```python
from build123d import *

# Parameters (mm, degrees)
SKETCH_1_R      = 4.402451684
SKETCH_1_R_2    = 1.6
EXTRUDE_1_DEPTH = 2
EXTRUDE_4_DEPTH = 8.8


with BuildPart() as part:
    # 草图1 → 凸台-拉伸1 (new body)
    # profile 1 of 2: a face of its own
    with BuildSketch(Plane.XY):
        Circle(SKETCH_1_R)
        Circle(SKETCH_1_R_2, mode=Mode.SUBTRACT)
    # profile 2 of 2: a face of its own
    with BuildSketch(Plane.XY):
        with BuildLine():
            ThreePointArc((4.402451684, 0), (0, -4.402451684), (-4.402451684, 0))
            Line((-4.402451684, 0), (-4.402451684, -12.835731795))
            Line((-4.402451684, -12.835731795), (4.402451684, -12.835731795))
            Line((4.402451684, -12.835731795), (4.402451684, 0))
        make_face()
    extrude(amount=EXTRUDE_1_DEPTH)

    # 草图4 → 凸台-拉伸4 (add)
    with BuildSketch(Plane.ZY.offset(4.402451684)):
        with BuildLine():
            ThreePointArc((6, -8.835731795), (4.828427125, -6.00730467), (2, -4.835731795))
            Line((2, -4.835731795), (2, -5.835731795))
            ThreePointArc((2, -5.835731795), (4.121320344, -6.714411452), (5, -8.835731795))
            ThreePointArc((5, -8.835731795), (4.121320344, -10.957052139), (2, -11.835731795))
            Line((2, -11.835731795), (2, -12.835731795))
            ThreePointArc((2, -12.835731795), (4.828427125, -11.66415892), (6, -8.835731795))
        make_face()
    extrude(amount=-EXTRUDE_4_DEPTH)


solid = part.part
```
Check sheet for the modelled part. Datum: model origin and axes. Units: mm. Give positions to 0.01 mm unless a question says otherwise; leave off trailing zeros. Loops run counter-clockwise (first coordinate to the right, second up) from the corner with the lowest first, then second, coordinate; pieces in that order, holes last. Notation, with made-up numbers: M 18,-30 L 49,-30 A12 cw 49,-18 Z; hole C 23,1 d8. An arc over 180 degrees is marked long. Answer as CSV lines item,"result".
Item 1: Draft check along Z on faces 1 (the face through (0, -4, 2)), 2 (the face through (-4.402, -7.8, 1.6)), 3 (the face through (0, -4, 0)). Enter one of: pulls with the +Z half, pulls with the -Z half, needs draft (parallel to the pull), parting line crosses it, or undercut.
Reply:
face 1,"undercut"
face 2,"needs draft"
face 3,"pulls with the -Z half"
Item 2: Sectioned sample at C-C, the plane y = -10.75. Enter the section's corners in (x, z), then the cut area to 3 significant figures.
Reply:
outline,"M -4.4,0 L 4.4,0 L 4.4,2 L -4.4,2 Z; M -4.4,4.31 L 4.4,4.31 L 4.4,5.51 L -4.4,5.51 Z"
area,"28.2 mm^2"
Item 3: Depth check by flat-ended pin: pin 1 Ø1 at (y, z) = (-6.5, 4.5) entering from +X; pin 2 Ø2.5 at (x, y) = (2, -3) entering from +Z; pin 3 Ø2 at (x, z) = (-2, 1.5) entering from +Y; pin 4 Ø1.9 at (x, y) = (0, 0) entering from -Z. Enter the tip coordinate at first touch or a pass-through.
Reply:
pin 1,"x = 4.4"
pin 2,"z = 2"
pin 3,"y = 4.29"
pin 4,"through"
Item 4: Scan lines: L1, parallel to Y at x = 0, z = 0.75; L2, parallel to Y at x = -0.75, z = 2.1; L3, parallel to Z at x = -1.25, y = 3.5. Record each from-to range of solid material in increasing order.
Reply:
L1,"-12.84 to -1.6, 1.6 to 4.4"
L2,"-12.83 to -11.83, -5.84 to -4.84"
L3,"0 to 2"
Item 5: Sectioned sample at D-D, the plane z = 4. Enter the section's corners in (x, y), then the cut area to 3 significant figures.
Reply:
outline,"M -4.4,-12.3 L 4.4,-12.3 L 4.4,-11.07 L -4.4,-11.07 Z; M -4.4,-6.6 L 4.4,-6.6 L 4.4,-5.37 L -4.4,-5.37 Z"
area,"21.6 mm^2"
Item 6: Sectioned sample at B-B, the plane z = 0.9. Enter the section's corners in (x, y).
Reply:
outline,"M -4.4,-12.84 L 4.4,-12.84 L 4.4,0 A4.4 ccw -4.4,0 Z; hole C 0,0 d3.2"
Item 7: Sectioned sample at A-A, the plane x = 0. Enter the section's corners in (y, z), then the cut area to 3 significant figures.
Reply:
outline,"M -12.84,0 L -1.6,0 L -1.6,2 L -4.84,2 A4 ccw -12.84,2 Z; M 1.6,0 L 4.4,0 L 4.4,2 L 1.6,2 Z; hole M -11.84,2 L -5.84,2 A3 ccw Z"
area,"39.1 mm^2"
